Part print with two shaded views. Sizes in mm from the minimum x, y, z corner. A direction names the side the tool comes from. Round coordinates to 2 decimals unless told otherwise and drop trailing zeros. Order: outer loops, then holes, each group sorted by start corner. A loop starts at its lowest first (then second) coordinate and runs counter-clockwise, first axis right, second up. Notation, with made-up numbers: M 15,39 L 58,39 A25 ccw 58,56 Z; hole C -16.5,61.5 d8. An arc over 180 degrees is marked long. Return JSON: item names as keys, results as strings. Group by question number.
Item 1: Slice it at C-C on y = 213.5. Write the cut outline in (x, z).
Item 2: Slice it at A-A on x = 116.5. Write the cut outline in (y, z).
Item 3: Slice it at B-B on z = 336.5. Write the cut outline in (x, y).
Item 4: Pin check, flat tip, straight feed: pin 1 Ø1 at (x, y) = (43.5, 206.5) entering from -Z. Stop position of the tip, or through.
Item 5: Probe line 1 along Y through (x, z) = (156, 414); line 2 along Z through (x, y) = (183.5, 370.5). List the from-to ranges inside material, lowest first.
Item 6: Which spindle directions (+Z, -Z, +X, -X, +Y, -Y) get a long thin tool onto all of the face, cutting with end or side? Do the marked faces 1 and 2. Say none if no direction does.
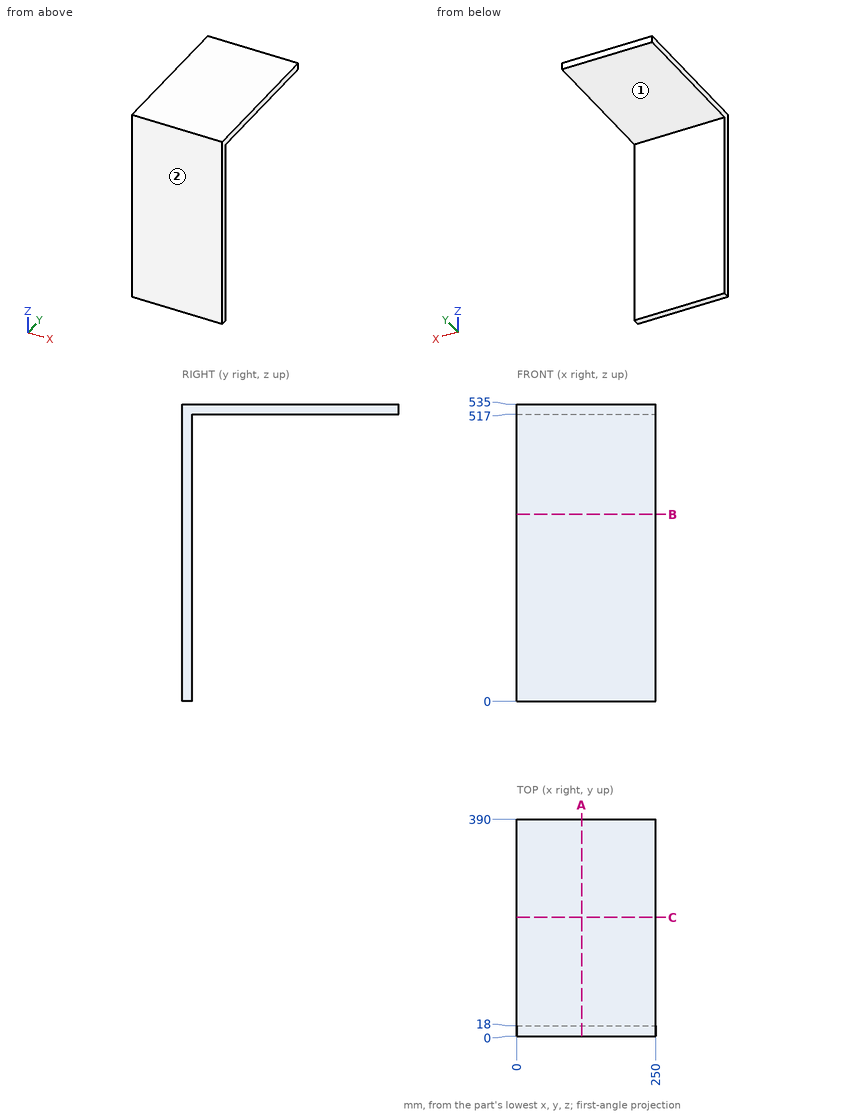
Output values:
{
 "1": {"outline": "M 0,517 L 250,517 L 250,535 L 0,535 Z"},
 "2": {"outline": "M 0,0 L 18,0 L 18,517 L 390,517 L 390,535 L 0,535 Z"},
 "3": {"outline": "M 0,0 L 250,0 L 250,18 L 0,18 Z"},
 "4": {"pin 1": "z = 517"},
 "5": {"line 1": "0 to 18", "line 2": "517 to 535"},
 "6": {"face 1": "-Z, +X, -X, +Y", "face 2": "+Z, -Z, +X, -X, -Y"}
}
